Source: three-view drawing plus pictorial views. Frame: mm from the lowest corner of the part. A direction names the side the tool comes from. Give positions to 0.01 mm unless a question says otherwise; leave off trailing zeros. Write each loop counter-clockwise with the first axis right and the second up, starting at its lowest first coordinate (ties: lowest second). Pieces come first, ordered by that corner, then holes.
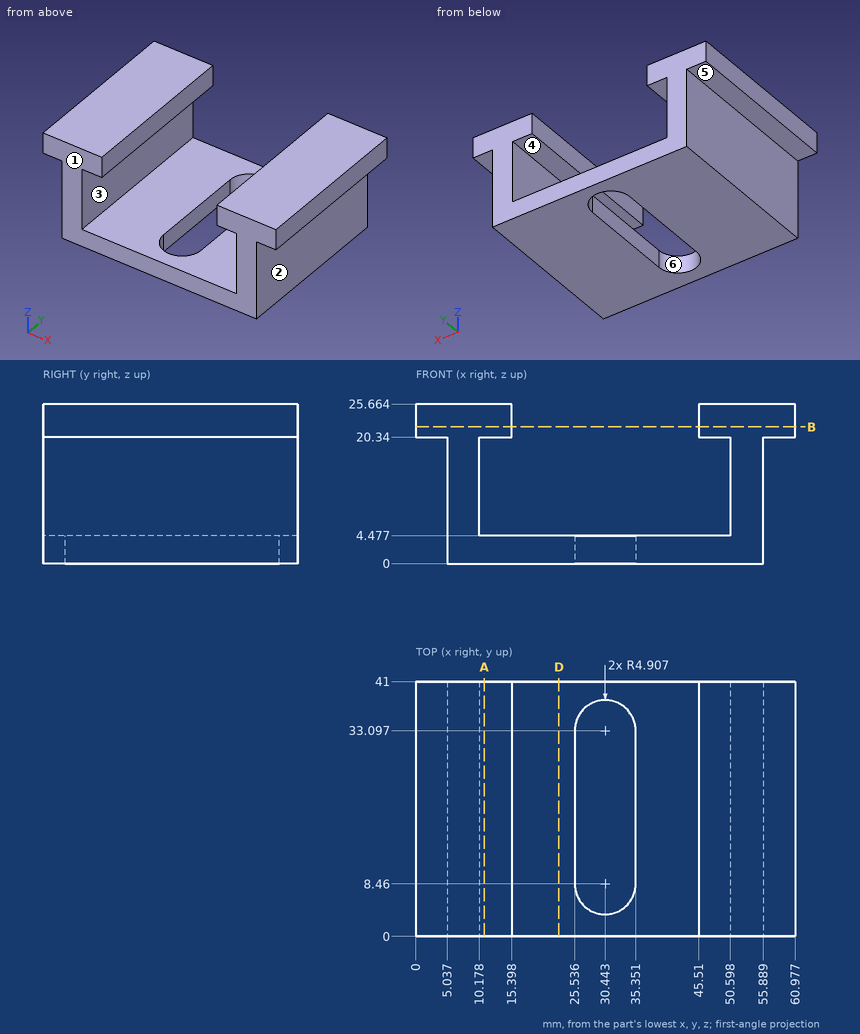
Q1. Section B-B on z = 22. Output: boundary loops of the cut face in (x, y), plus the area to 3 significant figures.
Filled sheet:
outline: (0, 0) - (15.4, 0) - (15.4, 41) - (0, 41) - close; (45.51, 0) - (60.98, 0) - (60.98, 41) - (45.51, 41) - close
area: 1,270 mm2
Q2. Ray query, line 1 along X through (y, z) = (10.5, 9.25); line 2 along Z through (x, y) = (46.5, 7.5) (1 decimal); line 3 along X through (y, z) = (30, 23.5). Return the intervals inside material, ascending.
Filled sheet:
line 1: x = 5.04 to 10.18, 50.6 to 55.89
line 2: z = 0 to 4.5, 20.3 to 25.7
line 3: x = 0 to 15.4, 45.51 to 60.98
Q3. Access query for the marked faces 4, 5 and 6. Directions: +Z, -Z, +X, -X, +Y, -Y. A direction counts if a zero-diameter tool reaches every point of the face in a straight line with its end or side. Return the directions, or none.
Filled sheet:
face 4: +Y, -Y
face 5: -Z, -X, +Y, -Y
face 6: +Z, -Z
Q4. Pin query (flat end, axial travel): P1, Ø10, axis at x = 24, z = 10, coming from the -Y side; P2, Ø4, axis at x = 1.5, y = 24.5, coming from the -Z side; P3, Ø5, axis at y = 17.5, z = 3.5, coming from the +X side; P4, Ø1.3, axis at y = 19.5, z = 2, coming from the -X side. Return the tip coordinate at first contact, or that it passes through.
Filled sheet:
P1: passes through
P2: stops at z = 20.34
P3: stops at x = 55.89
P4: stops at x = 5.04
Q5. Section D-D on x = 23. Output: boundary loops of the cut face in (y, z).
Filled sheet:
outline: (0, 0) - (41, 0) - (41, 4.48) - (0, 4.48) - close
Q6. Section A-A on x = 11. Output: boundary loops of the cut face in (y, z) (1 decimal).
Filled sheet:
outline: (0, 0) - (41, 0) - (41, 4.5) - (0, 4.5) - close; (0, 20.3) - (41, 20.3) - (41, 25.7) - (0, 25.7) - close
Q7. Pull-direction query (X, two-part tool) for the marked faces 1, 2 and 3; classes: released by +X, released by -X, zero draft, split by the parting line, or undercut.
Filled sheet:
face 1: zero draft
face 2: released by +X
face 3: undercut
